Build history of the part. All positions in model axes, mm. A direction names the side the tool comes from. Round coordinates to 2 decimals unless told otherwise and drop trailing zeros. Order: outer loops, then holes, each group sorted by start corner. A loop starts at its lowest first (then second) coordinate and runs counter-clockwise, first axis right, second up. Notation, with made-up numbers: (76.25, 74.25) -> (132.25, 74.25) arc R19 ccw to (132.25, 96.25) -> close; hole circle Ø7 at (-23, 59). An arc over 180 degrees is marked (long way). Answer as a JSON object with one key per item and string values.
Autodesk Inventor part; units mm, degrees
ref_plane "Work Plane1" through (104.775, 0, 0) normal (0, 0, -1) x (1, 0, 0)
ref_plane "YZ Plane" through (0, 0, 0) normal (1, 0, 0) x (0, 1, 0)
ref_plane "XZ Plane" through (0, 0, 0) normal (0, 1, 0) x (-1, 0, 0)
sketch "Esquisse1" plane through (0, 0, 0) normal (0, 0, 1) x (1, 0, 0)
  line L0 (10, 0) -> (10, 2.5)
  line L1 (10, 2.5) -> (5.6, 2.5)
  line L2 (5.6, 2.5) -> (5.1092, 2.5)
  line L3 (0, 4.715) -> (0, 1.7321)
  line L4 (0, 1.7321) -> (2.14, 1.7321)
  line L5 (2.14, 1.7321) -> (3.14, 0)
  line L6 (3.14, 0) -> (10, 0)
  line L7 (0, 4.715) -> (0.885, 4.715)
  line L8 (0.885, 4.715) -> (3.1, 2.5)
  line L9 (5.1092, 2.5) -> (3.1, 2.5)
  line L10 (5.6, 2.5) -> (3.1, 2.5) construction
  line L11 (3.1, 2.5) -> (3.1, 2.5)
  line L12 (-2, 0) -> (12, 0)
  line L13 (0, -0.943) -> (0, 5.658)
  dimension "d0" = 10
  dimension "d1" = 4.4
  dimension "d2" = 2.14
  dimension "d3" = 5
  dimension "d6" = 3.1
  dimension "d7" = 45
  dimension "d8" = 3.4641
  dimension "d9" = 60
  dimension "d10" = 9.43
  dimension "d11" = 5
  dimension "d12" = 0.4908
revolve "Corps" add sketch "Esquisse1" angle 360 about axis through (3.14, 0, 0) along (1, 0, 0) contours L6 L5 L4 L3 L7 L8 L9 L2 L1 L0
sketch "Esquisse2" plane through (0, 0, 0) normal (-1, 0, 0) x (0, 0, 1)
  circle A0 centre (0, 0) radius 1.7321
  line L0 (0, -6.601) -> (0, 6.601)
  line L1 (-6.601, 0) -> (6.601, 0)
  line L2 (1.7321, 0) -> (0.866, -1.5)
  line L3 (0.866, -1.5) -> (-0.866, -1.5)
  line L4 (-0.866, -1.5) -> (-1.7321, 0)
  line L5 (-1.7321, 0) -> (-0.866, 1.5)
  line L6 (-0.866, 1.5) -> (0.866, 1.5)
  line L7 (0.866, 1.5) -> (1.7321, 0)
  point P0 (0, 1.7321)
extrude "Rainure" add sketch "Esquisse2" against normal up to next contours L7 A0 | A0 L2 | L6 L0 A0 | A0 L0 L3 | L0 L6 A0 | A0 L3 L0 | L4 A0 | A0 L5
thread "Filetage"
chamfer "Chanfrein1" distance 0.4908 distance2 0.4908 1 edges at (10, -2.5, 0) measured on face at (10, 0.4809, 1.5312)
ref_plane "Work Plane1" through (104.775, 0, 0) normal (0, 0, -1) x (1, 0, 0)
equation "\"d15\" = GEL"
equation "\"d17\" = -0.5 * SPD + 0.5 * GD"
equation "\"d18\" = GUL"
equation "\"d0\" = NLG"
equation "\"d1\" = GEL"
equation "\"d2\" = INTI"
equation "\"d3\" = GD"
equation "\"d6\" = KOH"
equation "\"d7\" = 0.5 * SEWI"
equation "\"d8\" = 1.1547 * SW"
equation "\"d10\" = KOD"
equation "\"d11\" = BDM"
equation "\"d12\" = GAL"
equation "\"NLG\" = 10"
equation "\"INTI\" = 2.14"
equation "\"GEL\" = 4.4"
equation "\"GAL\" = 0.61345 * PTC"
equation "\"KOH\" = 3.1"
equation "\"KOD\" = 9.43"
equation "\"GUL\" = 0.61345 * PTC"
equation "\"SPD\" = NND - 1.2269 * PTC"
equation "\"BDM\" = NND"
equation "\"GD\" = NND"
equation "\"SEWI\" = 90deg"
equation "\"SW\" = 3"
equation "\"TOA\" = 30deg"
equation "\"GD1\" = THREADDIA - 1.2269 * PTC"
equation "\"EPV\" = 5.6"
equation "\"THREADDIA\" = 5"
equation "\"PTC\" = 0.8"
equation "\"NND\" = 5"
equation "\"E0\" = 3.47"
equation "\"THREADDESC\" = 1.2345"
properties part number "ISO 10642 - M5 x  10" material "Acier"
1) Which spindle directions (+Z, -Z, +X, -X, +Y, -Y) get a long thin tool onto all of the face, cutting with end or side? Do faces 4 (the face through (0.449, -0.614, 4.675)), 5 (the face through (6.26, -0.54, 2.44)), 6 (the face through (1, -1.5, 0)). Say none if no direction does.
Checked values:
{"face 4": "+X, -X", "face 5": "+X", "face 6": "-X"}
2) Pull direction Z, two halves, no side cores. Call faces 1 (the face through (1.121, -0.761, -1.293)), 2 (the face through (2.96, -2.09, 1.61)), 3 (the face through (0, 0, 2)): pulls with the +Z half, pulls with the -Z half, needs draft (parallel to the pull), parting line crosses it, or undercut.
Checked values:
{"face 1": "undercut", "face 2": "parting line crosses it", "face 3": "needs draft"}
3) Cut at B-B, the plane x = 2.75. Give the cut face in (y, z), plus the area to 3 significant figures.
Checked values:
{"outline": "circle Ø5.7 at (0, 0); hole circle Ø1.35 at (0, 0)", "area": "24.1 mm²"}
4) Cut at A-A, the plane x = 7.25. Give the cut face in (y, z).
Checked values:
{"outline": "circle Ø5 at (0, 0)"}
5) Probe L1, parallel to X at y = -2, z = 0.75; L2, parallel to Z at x = 2, y = 2; L3, parallel to X at y = -1, z = 1. List the from-to ranges inside material, lowest first. Write a range as from..to.
Checked values:
{"L1": "x = 0..9.87", "L2": "z = -2.99..2.99", "L3": "x = 2.32..10"}
6) Flat gauge pins, fed straight in: pin 1 Ø1.4 at (x, z) = (1, -0.5) entering from +Y (3 decimals); pin 2 Ø1 at (x, z) = (3, -2) entering from -Y; pin 3 Ø2 at (x, z) = (4.5, 3) entering from +Y; pin 4 Ø2 at (x, y) = (5.5, 1) entering from +Z. Where does each tip first touch, or does it go through?
Checked values:
{"pin 1": "stops at y = 4.715", "pin 2": "stops at y = -2.48", "pin 3": "stops at y = 1.5", "pin 4": "stops at z = 2.5"}
